```python
from build123d import *

# Parameters (mm, degrees)
SKETCH1_R           = 8.75
SKETCH1_R_2         = 7.6
BOSS_EXTRUDE1_DEPTH = 7.5
SKETCH1_2_R         = 7.6
BOSS_EXTRUDE2_DEPTH = 2.5
SKETCH2_R           = 6.25
SKETCH2_R_2         = 3.75
BOSS_EXTRUDE3_DEPTH = 4.5
CUT_EXTRUDE1_START  = -4.5
SKETCH3_R           = 3.75
CUT_EXTRUDE1_DEPTH  = 4.5


with BuildPart() as part:
    # Sketch1 → Boss-Extrude1 (new body)
    with BuildSketch(Plane(origin=(0, 0, 0), x_dir=(1, 0, 0), z_dir=(0, 1, 0))):
        with Locations(Location((0, 0, 0), (0, 0, 270))):
            Circle(SKETCH1_R)
        with Locations(Location((0, 0, 0), (0, 0, 270))):
            Circle(SKETCH1_R_2, mode=Mode.SUBTRACT)
    extrude(amount=BOSS_EXTRUDE1_DEPTH)

    # Sketch1_2 → Boss-Extrude2 (add)
    with BuildSketch(Plane(origin=(0, 0, 0), x_dir=(1, 0, 0), z_dir=(0, 1, 0))):
        with Locations(Location((0, 0, 0), (0, 0, 270))):
            Circle(SKETCH1_2_R)
    extrude(amount=BOSS_EXTRUDE2_DEPTH)

    # Sketch2 → Boss-Extrude3 (add)
    with BuildSketch(Plane.XZ):
        with Locations(Location((0, 0, 0), (0, 0, 90))):
            Circle(SKETCH2_R)
        with Locations(Location((0, 0, 0), (0, 0, 270))):
            Circle(SKETCH2_R_2, mode=Mode.SUBTRACT)
    extrude(amount=BOSS_EXTRUDE3_DEPTH)

    # Sketch3 → Cut-Extrude1 (cut)
    with BuildSketch(Plane.XZ.offset(CUT_EXTRUDE1_START)):
        with Locations(Location((0, 0, 0), (0, 0, 90))):
            Circle(SKETCH3_R)
    extrude(amount=CUT_EXTRUDE1_DEPTH, mode=Mode.SUBTRACT)

    # Sketch4 → Revolve1 (revolve)
    with BuildSketch(Plane.XY, mode=Mode.PRIVATE) as revolve1_sk:
        Polygon((2.25, -1.5), (3.75, -1.5), (3.75, 2.5), align=None)
    revolve(revolve1_sk.sketch.rotate(Axis((0, 6.48863082, 0), (0, -1, 0)), 90), axis=Axis((0, 6.48863082, 0), (0, -1, 0)))


solid = part.part
```
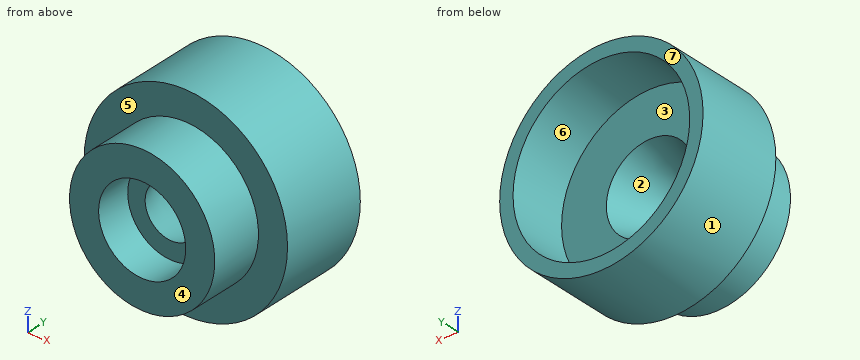
Source: CAD feature listing. Evaluate the final solid. Frame: model axes, mm. Face numbers are marked on the shaded views. A direction names the side the tool comes from. Coordinates: 2 decimals unless noted, no trailing zeros. Loops run counter-clockwise (first coordinate to the right, second up) from the corner with the lowest first, then second, coordinate; pieces in that order, holes last. Notation, with made-up numbers: M 31,20.25 L 51,20.25 A33 cw 51,50.25 Z; hole C 19.5,64.5 d3. An arc over 180 degrees is marked long. Put each result on its own line as item: value. Start each with the question number.
1) Pull-direction query (Z, two-part tool) for the marked faces 1, 2, 3 and 4; classes: pulls with the +Z half, pulls with the -Z half, needs draft (parallel to the pull), parting line crosses it, or undercut.
2) Cut plane B-B on x = 0. Return the cut outline in (y, z).
3) Reachability of the marked faces 5, 6 and 7 from +Z, -Z, +X, -X, +Y, -Y: full face, straight path, thin tool, end or side. Return the list, or none.
4) Ray query, L1, parallel to X at y = 4.05, z = 0; L2, parallel to X at y = -2.55, z = 0. Return the intervals inside material, ascending. Write a range as from..to.
5) Cut plane A-A on z = 0. Return the cut outline in (x, y), then the cut area to 3 significant figures.
6) Cut plane C-C on y = 6. Return the cut outline in (x, z), then the cut area to 3 significant figures.
7) Contact query for flat-ended pins moving along their axis: pin 1 Ø1 at (y, z) = (5.5, -3) entering from +X; pin 2 Ø5 at (y, z) = (0.5, 3) entering from +X; pin 3 Ø1.5 at (x, z) = (-7, 0) entering from +Y; pin 4 Ø3 at (y, z) = (0.5, 2) entering from -X. Output: stop coordinate, or through.
8) Cut plane D-D on x = -5.5. Return the cut outline in (y, z) (3 decimals).
The answers:
1. face 1: parting line crosses it
1. face 2: undercut
1. face 3: undercut
1. face 4: needs draft
2. outline: M -4.5,-6.25 L 0,-6.25 L 0,-8.75 L 7.5,-8.75 L 7.5,-7.6 L 2.5,-7.6 L 2.5,-3.75 L -1.5,-2.25 L -1.5,-3.75 L -4.5,-3.75 Z; M -4.5,3.75 L -1.5,3.75 L -1.5,2.25 L 2.5,3.75 L 2.5,7.6 L 7.5,7.6 L 7.5,8.75 L 0,8.75 L 0,6.25 L -4.5,6.25 Z
3. face 5: -Y
3. face 6: +Y
3. face 7: +Z, -Z, +X, -X, +Y
4. L1: x = -8.75..-7.6, 7.6..8.75
4. L2: x = -6.25..-3.75, 3.75..6.25
5. outline: M -8.75,0 L -6.25,0 L -6.25,-4.5 L -3.75,-4.5 L -3.75,-1.5 L -2.25,-1.5 L -3.75,2.5 L -7.6,2.5 L -7.6,7.5 L -8.75,7.5 Z; M 2.25,-1.5 L 3.75,-1.5 L 3.75,-4.5 L 6.25,-4.5 L 6.25,0 L 8.75,0 L 8.75,7.5 L 7.6,7.5 L 7.6,2.5 L 3.75,2.5 Z
5. area: 65.0 mm²
6. outline: C 0,0 d17.5; hole C 0,0 d15.2
6. area: 59.1 mm²
7. pin 1: stops at x = 8.39
7. pin 2: stops at x = 8.74
7. pin 3: stops at y = 7.5
7. pin 4: stops at x = -8.74
8. outline: M -4.5,-2.969 L 0,-2.969 L 0,-6.805 L 7.5,-6.805 L 7.5,-5.245 L 2.5,-5.245 L 2.5,5.245 L 7.5,5.245 L 7.5,6.805 L 0,6.805 L 0,2.969 L -4.5,2.969 Z
